from build123d import *

# Parameters (mm, degrees)
SKETCH1_R           = 4
BOSS_EXTRUDE1_DEPTH = 30
SKETCH2_R           = 1.7
CUT_EXTRUDE1_DEPTH  = 18


with BuildPart() as part:
    # Sketch1 → Boss-Extrude1 (new body)
    with BuildSketch(Plane(origin=(0, 0, 0), x_dir=(1, 0, 0), z_dir=(0, 1, 0))):
        Polygon((-7, 10), (7, 10), (8, 11), (16, 11), (17, 10), (17, 5), (15, 3), (15, -7), (7.091285061, -7), (3.091285061, -11), (-3.091285061, -11), (-7.091285061, -7), (-15, -7), (-15, 3), (-17, 5), (-17, 10), (-16, 11), (-8, 11), align=None)
        with Locations(Location((0, 0, 0), (0, 0, 270))):
            Circle(SKETCH1_R, mode=Mode.SUBTRACT)
    extrude(amount=BOSS_EXTRUDE1_DEPTH)

    # Sketch2 → Cut-Extrude1 (cut)
    with BuildSketch(Plane.XY.offset(7)):
        with Locations((12, 24)):
            Circle(SKETCH2_R)
        with Locations((-12, 24)):
            Circle(SKETCH2_R)
        with Locations((-12, 6)):
            Circle(SKETCH2_R)
        with Locations((12, 6)):
            Circle(SKETCH2_R)
    extrude(amount=-CUT_EXTRUDE1_DEPTH, mode=Mode.SUBTRACT)


solid = part.part
Work out the finished part from the listing and answer in its coordinate system (mm). A direction names the side the tool comes from. Round coordinates to 2 decimals unless told otherwise and drop trailing zeros. Write each loop counter-clockwise with the first axis right and the second up, starting at its lowest first coordinate (ties: lowest second). Pieces come first, ordered by that corner, then holes.
1) Given pin 1 Ø1 at (y, z) = (6.5, -0.5) entering from -X; pin 2 Ø4 at (x, y) = (-10.5, 12) entering from +Z; pin 3 Ø1 at (x, y) = (-4, 21.5) entering from -Z, each flat-ended and moving along its own axis, determine where each tip first touches the part or whether it passes through.
2) A cutting plane is placed at D-D (x = 0). Give the vertices of the cut face in (y, z), plus the area to 3 significant figures.
3) A cutting plane is placed at B-B (x = -12). Give the vertices of the cut face in (y, z), plus the area to 3 significant figures.
4) A cutting plane is placed at A-A (z = 0). Give the vertices of the cut face in (x, y), plus the area to 3 significant figures.
5) Straight lines are drawn through the part: line 1 (Y direction, x = 12, z = -4); line 2 (X direction, y = 19, z = 0); line 3 (Z direction, x = -14, y = 11.75). For each, find the intervals that lie inside material, in ascending order.
6) A cutting plane is placed at C-C (y = 6). Give the vertices of the cut face in (x, z), plus the area to 3 significant figures.
7) A tool of negligible diameter and unlimited length cuts with its end or side. For faces 4 (the flat face through (16.5, 14.8, -10.5)), 5 (the flat face through (-11, 15, 7)), 6 (the flat face through (-7.5, 14.8, -10.5)), from which of +Z, -Z, +X, -X, +Y, -Y can it reach the whole face along a straight path? Write none if from no direction.
8) The mould has two halves that part along Z. Classify faces 1 (the flat face through (-16.5, 14.8, -10.5)), 2 (the flat face through (-15, 15, 2)), 3 (the cylindrical face through (-3.905, 14.79, -0.867)): pulls with the +Z half, pulls with the -Z half, needs draft (parallel to the pull), parting line crosses it, or undercut.
Completed:
1. pin 1: stops at x = -15
1. pin 2: stops at z = 7
1. pin 3: stops at z = -10
2. outline: (0, -10) - (30, -10) - (30, -4) - (0, -4) - close; (0, 4) - (30, 4) - (30, 11) - (0, 11) - close
2. area: 390 mm2
3. outline: (0, -11) - (4.3, -11) - (4.3, 7) - (0, 7) - close; (7.7, -11) - (22.3, -11) - (22.3, 7) - (7.7, 7) - close; (25.7, -11) - (30, -11) - (30, 7) - (25.7, 7) - close
3. area: 418 mm2
4. outline: (-15, 0) - (-4, 0) - (-4, 30) - (-15, 30) - close; (4, 0) - (15, 0) - (15, 30) - (4, 30) - close; hole circle Ø3.4 at (-12, 6); hole circle Ø3.4 at (-12, 24); hole circle Ø3.4 at (12, 6); hole circle Ø3.4 at (12, 24)
4. area: 624 mm2
5. line 1: y = 0 to 4.3, 7.7 to 22.3, 25.7 to 30
5. line 2: x = -15 to -4, 4 to 15
5. line 3: z = -11 to 7
6. outline: (-17, -10) - (-16, -11) - (-13.7, -11) - (-13.7, 7) - (-15, 7) - (-15, -3) - (-17, -5) - close; (-10.3, -11) - (-8, -11) - (-7, -10) - (7, -10) - (8, -11) - (10.3, -11) - (10.3, 7) - (7.09, 7) - (3.09, 11) - (-3.09, 11) - (-7.09, 7) - (-10.3, 7) - close; (13.7, -11) - (16, -11) - (17, -10) - (17, -5) - (15, -3) - (15, 7) - (13.7, 7) - close; hole circle Ø8 at (0, 0)
6. area: 420 mm2
7. face 4: -Z, +X, +Y, -Y
7. face 5: +Z, -X, +Y, -Y
7. face 6: -Z, +Y, -Y
8. face 1: pulls with the -Z half
8. face 2: needs draft
8. face 3: undercut
